Verification items for the finished model (mm, model axes). A direction names the side the tool comes from. Give positions to 0.01 mm unless a question says otherwise; leave off trailing zeros. Write each loop counter-clockwise with the first axis right and the second up, starting at its lowest first coordinate (ties: lowest second). Pieces come first, ordered by that corner, then holes. Notation, with made-up numbers: (15, 2) -> (44, 2) arc R15 cw to (44, 27) -> close; hole circle Ø4 at (61, -16). An arc over 180 degrees is marked (long way). Answer as CSV lines item,"result".
```python
from build123d import *

# Parameters (mm, degrees)
F1_DEPTH      = 10
F1_DEPTH_BACK = 10
F3_DEPTH      = 10.001
F5_DEPTH      = 5.5
F6_R          = 1.395
F7_DEPTH      = 1.5
F8_R          = 5.5
F9_DEPTH      = 2
F10_R         = 4.25
F11_DEPTH     = 110.584302492
F12_R         = 1.5
F13_R         = 20


with BuildPart() as f1:
    # F0 (on Front) → F1 (new body, two sides)
    with BuildSketch(Plane.XZ) as f1_sk:
        Polygon((30, 51.9615242271), (0, 0), (130, 0), (130, 10), (82.6794919243, 10), (60.9400542571, 22.5512701892), (62.9400542571, 26.0153718044), (45.6195461814, 36.0153718044), (43.6195461814, 32.5512701892), (26.2990381057, 42.5512701892), (31.2990381057, 51.2115242271), align=None)
        with BuildLine():
            ThreePointArc((23.0490381057, 36.9221050646), (26.0850698991, 39.2517341961), (29.8791651246, 38.7522320835))
            Line((29.8791651246, 38.7522320835), (78.2416697508, 10.8301270189))
            ThreePointArc((78.2416697508, 10.8301270189), (80.5712988822, 5.2059047745), (75.7416697508, 1.5))
            Line((75.7416697508, 1.5), (27.4019237886, 1.5))
            Line((27.4019237886, 1.5), (13.1291651246, 9.7403810568))
            ThreePointArc((13.1291651246, 9.7403810568), (10.7995359932, 12.7764128502), (11.2990381057, 16.5705080757))
            Line((11.2990381057, 16.5705080757), (23.0490381057, 36.9221050646))
        make_face(mode=Mode.SUBTRACT)
    extrude(amount=F1_DEPTH)
    extrude(f1_sk.sketch, amount=-F1_DEPTH_BACK)

    # F2 (on face) → F3 (cut, through all)
    with BuildSketch(Plane.XY.offset(10)):
        with BuildLine():
            Line((98, 5), (130, 5))
            Line((130, 5), (130, 10))
            Line((130, 10), (95, 10))
            Line((95, 10), (95, 8))
            ThreePointArc((95, 8), (95.8786796564, 5.8786796564), (98, 5))
        make_face()
        with BuildLine():
            Line((130, 0), (130, 3))
            Line((130, 3), (113, 3))
            ThreePointArc((113, 3), (110.8786796564, 2.1213203436), (110, 0))
            ThreePointArc((110, 0), (110.8786796564, -2.1213203436), (113, -3))
            Line((113, -3), (130, -3))
            Line((130, -3), (130, 0))
        make_face()
        with BuildLine():
            ThreePointArc((98, -5), (95.8786796564, -5.8786796564), (95, -8))
            Line((95, -8), (95, -10))
            Line((95, -10), (130, -10))
            Line((130, -10), (130, -5))
            Line((130, -5), (98, -5))
        make_face()
    extrude(amount=-F3_DEPTH, mode=Mode.SUBTRACT)

    # F4 (on face) → F5 (cut, through all)
    with BuildSketch(Plane(origin=(27, 0, 46.7653718044), x_dir=(0.8660254038, 0, -0.5), z_dir=(0.5, 0, 0.8660254038))):
        with BuildLine():
            Line((28, -4), (35, -4))
            ThreePointArc((35, -4), (39, 0), (35, 4))
            Line((35, 4), (28, 4))
            ThreePointArc((28, 4), (24, 0), (28, -4))
        make_face()
    extrude(amount=-F5_DEPTH, mode=Mode.SUBTRACT)

    # F6 (on face) → F7 (cut, through all)
    with BuildSketch(Plane(origin=(0, 0, 0), x_dir=(0, -1, 0), z_dir=(-0.8660254038, 0, 0.5))):
        with Locations((-5, 39)):
            Circle(F6_R)
        with Locations((5, 39)):
            Circle(F6_R)
        with Locations((-5, 32)):
            Circle(F6_R)
        with Locations((5, 32)):
            Circle(F6_R)
        with Locations((-5, 25)):
            Circle(F6_R)
        with Locations((5, 25)):
            Circle(F6_R)
    extrude(amount=-F7_DEPTH, mode=Mode.SUBTRACT)

    # F8 (on face) → F9 (cut)
    with BuildSketch(Plane(origin=(0, 0, 0), x_dir=(0, -1, 0), z_dir=(-0.8660254038, 0, 0.5))):
        with Locations((0, 7.5)):
            Circle(F8_R)
    extrude(amount=-F9_DEPTH, mode=Mode.SUBTRACT)

    # F10 (on face) → F11 (cut, through all)
    with BuildSketch(Plane(origin=(1.7320508076, 0, -1), x_dir=(0, -1, 0), z_dir=(-0.8660254038, 0, 0.5))):
        with Locations((0, 7.5)):
            Circle(F10_R)
    extrude(amount=-F11_DEPTH, mode=Mode.SUBTRACT)

    # F12
    f12_edges = [f1.edges().sort_by_distance(p)[0] for p in [
        (26.299038, 0, 42.55127),
        (60.940054, 0, 22.55127),
        (27.401924, 0, 1.5),
        (43.619546, 0, 32.55127),
    ]]
    fillet(f12_edges, radius=F12_R)

    # F13
    f13_edges = [f1.edges().sort_by_distance(p)[0] for p in [
        (82.679492, 0, 10),
    ]]
    fillet(f13_edges, radius=F13_R)


solid = f1.part
```
1) Depth check by flat-ended pin: pin 1 (5 mm diameter, centred on x = 120, z = 3, fed in from -Y); pin 2 (3 mm diameter, centred on x = 116, z = 3.5, fed in from +Y); pin 3 (6 mm diameter, centred on y = 7, z = 19, fed in from +X); pin 4 (1.5 mm diameter, centred on x = 47, y = 5.5, fed in from -Z). Enter the tip coordinate at first touch or a pass-through.
Reported:
pin 1,"y = -5"
pin 2,"y = 5"
pin 3,"x = 72.29"
pin 4,"z = 0"
2) Scan lines: line 1 along Z through (x, y) = (28, -3.75); line 2 along X through (y, z) = (-2, 11.5); line 3 along Z through (x, y) = (66.5, 5). Record each from-to range of solid material in increasing order.
Reported:
line 1,"0 to 1.5, 39.38 to 41.57, 45.5 to 48.5"
line 2,"6.64 to 11.34, 77.08 to 80.44"
line 3,"0 to 1.5, 17.61 to 19.34"
3) Section check C-C (x = 96.5). Record the boundary of the cut face in (y, z).
Reported:
outline,"(-5.4, 0) -> (5.4, 0) -> (5.4, 10) -> (-5.4, 10) -> close"
4) Tool access check on faces 4 (the cylindrical face through (10.814, -0.14, 12.723)), 5 (the flat face through (114, -5, 5)), 6 (the flat face through (3.254, 0.026, 1.636)). Record the directions out of +Z, -Z, +X, -X, +Y, -Y that give a thin tool (end or side, any length) a straight path to the whole face; none if there is none.
Reported:
face 4,"+Y, -Y"
face 5,"+Z, -Z, +X, -Y"
face 6,"none"
5) Section check A-A (x = 64.5). Record the boundary of the cut face in (y, z), and give its area (3 significant figures).
Reported:
outline,"(-10, 0) -> (10, 0) -> (10, 1.5) -> (-10, 1.5) -> close; (-10, 18.76) -> (10, 18.76) -> (10, 20.5) -> (-10, 20.5) -> close"
area,"64.6 mm²"
6) Section check B-B (z = 46.5). Record the boundary of the cut face in (x, y), and give its area (3 significant figures).
Reported:
outline,"(26.85, -10) -> (28.58, -10) -> (28.58, 10) -> (26.85, 10) -> close"
area,"34.6 mm²"
7) Draft check along Z on faces 1 (the flat face through (62.306, -0.14, 24.918)), 2 (the flat face through (44, 10, 1)), 3 (the flat face through (54.401, -4.584, 30.945)). Enter one of: +Z half, -Z half, draft (parallel to the pull), parting line (faces both ways), or undercut.
Reported:
face 1,"undercut"
face 2,"draft"
face 3,"+Z half"
